Geometry check sheet. Reference: the model listing, model coordinates, mm. Round coordinates to 2 decimals unless told otherwise and drop trailing zeros. Order: outer loops, then holes, each group sorted by start corner. A loop starts at its lowest first (then second) coordinate and runs counter-clockwise, first axis right, second up.
(1) Cross-section at C-C on y = 17.5. Enter the section's corners in (x, z).
(2) Cross-section at A-A on y = -17.5. Enter the section's corners in (x, z).
(3) Cross-section at B-B on x = 48.14. Enter the section's corners in (y, z), and give its area (3 significant figures).
(4) Gauge pin test, flat end, axial feed: P1, Ø4, axis at x = 48.14, y = -17.5, coming from the -Z side. Record the tip position at first contact, or that the pin passes through.
(5) Thickness scan on L1, parallel to Y at x = 48.14, z = -0.45; L2, parallel to Y at x = -45.64, z = 0; L3, parallel to X at y = 19, z = -0.75. Record the ranges inside material, lowest first.
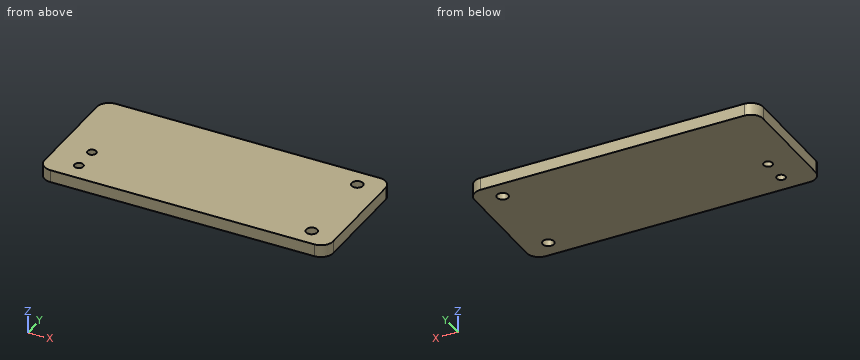
from build123d import *

# Parameters (mm, degrees)
F0_W     = 116.28
F0_H     = 50
F0_R     = 1.75
F0_R_2   = 2.25
F1_DEPTH = 2.5
F2_R     = 5


with BuildPart() as f1:
    # F0 (on Top) → F1 (new body, symmetric)
    with BuildSketch(Plane.XY):
        Rectangle(F0_W, F0_H)
        with Locations((-45.64, -17.5)):
            Circle(F0_R, mode=Mode.SUBTRACT)
        with Locations((-45.64, -7.5)):
            Circle(F0_R, mode=Mode.SUBTRACT)
        with Locations((48.14, -17.5)):
            Circle(F0_R_2, mode=Mode.SUBTRACT)
        with Locations((48.14, 17.5)):
            Circle(F0_R_2, mode=Mode.SUBTRACT)
    extrude(amount=F1_DEPTH, both=True)

    # F2
    f2_edges = [f1.edges().sort_by_distance(p)[0] for p in [
        (-58.14, -25, 0),
        (58.14, -25, 0),
        (58.14, 25, 0),
        (-58.14, 25, 0),
    ]]
    fillet(f2_edges, radius=F2_R)


solid = f1.part
Found:
1. outline: (-58.14, -2.5) - (45.89, -2.5) - (45.89, 2.5) - (-58.14, 2.5) - close; (50.39, -2.5) - (58.14, -2.5) - (58.14, 2.5) - (50.39, 2.5) - close
2. outline: (-58.14, -2.5) - (-47.39, -2.5) - (-47.39, 2.5) - (-58.14, 2.5) - close; (-43.89, -2.5) - (45.89, -2.5) - (45.89, 2.5) - (-43.89, 2.5) - close; (50.39, -2.5) - (58.14, -2.5) - (58.14, 2.5) - (50.39, 2.5) - close
3. outline: (-25, -2.5) - (-19.75, -2.5) - (-19.75, 2.5) - (-25, 2.5) - close; (-15.25, -2.5) - (15.25, -2.5) - (15.25, 2.5) - (-15.25, 2.5) - close; (19.75, -2.5) - (25, -2.5) - (25, 2.5) - (19.75, 2.5) - close
3. area: 205 mm2
4. P1: passes through
5. L1: y = -25 to -19.75, -15.25 to 15.25, 19.75 to 25
5. L2: y = -25 to -19.25, -15.75 to -9.25, -5.75 to 25
5. L3: x = -58.14 to 46.46, 49.82 to 58.14
